```python
from build123d import *

# Parameters (mm, degrees)
EXTRUDE_1_DEPTH     = 20
OTHER_START         = 15
OTHER_1_OUTLINE_R   = 4.05
OTHER_1_DEPTH       = 20
CUT_EXTRUDE_1_DEPTH = 10


# Read off the part's stored shape, not the designer's step: 高级异型孔1
with BuildPart() as part:
    # 草图3 → 凸台-拉伸1 (new body)
    with BuildSketch(Plane.XY.offset(15)):
        with BuildLine():
            Line((26.887488657, 8.75), (45, 8.75))
            Line((45, 8.75), (45, 23.25))
            Line((45, 23.25), (26.887488657, 23.25))
            ThreePointArc((26.887488657, 23.25), (20, 26), (13.112511343, 23.25))
            Line((13.112511343, 23.25), (-5, 23.25))
            Line((-5, 23.25), (-5, 8.75))
            Line((-5, 8.75), (13.112511343, 8.75))
            ThreePointArc((13.112511343, 8.75), (20, 6), (26.887488657, 8.75))
        make_face()
    extrude(amount=EXTRUDE_1_DEPTH)

    # 高级异型孔1 outline → 高级异型孔1 (cut)
    with BuildSketch(Plane.XY.offset(OTHER_START)):
        with Locations((20, 16)):
            Circle(OTHER_1_OUTLINE_R)
    extrude(amount=OTHER_1_DEPTH, mode=Mode.SUBTRACT)

    # 草图6 → 切除-拉伸1 (cut)
    with BuildSketch(Plane.XY.offset(35)):
        with BuildLine():
            Line((-5, 15.5), (-5, 17.25))
            Line((-5, 17.25), (10, 17.25))
            Line((10, 17.25), (10, 15.5))
            Line((10, 15.5), (7, 15.5))
            ThreePointArc((7, 15.5), (6.25, 14.75), (5.5, 15.5))
            ThreePointArc((5.5, 15.5), (4.75, 16.25), (4, 15.5))
            ThreePointArc((4, 15.5), (3.25, 14.75), (2.5, 15.5))
            ThreePointArc((2.5, 15.5), (1.75, 16.25), (1, 15.5))
            ThreePointArc((1, 15.5), (0.25, 14.75), (-0.5, 15.5))
            ThreePointArc((-0.5, 15.5), (-1.25, 16.25), (-2, 15.5))
            ThreePointArc((-2, 15.5), (-2.75, 14.75), (-3.5, 15.5))
            ThreePointArc((-3.5, 15.5), (-4.25, 16.25), (-5, 15.5))
        make_face()
        with BuildLine():
            Line((45, 17.25), (30, 17.25))
            Line((30, 17.25), (30, 15.5))
            Line((30, 15.5), (33, 15.5))
            ThreePointArc((33, 15.5), (33.75, 14.75), (34.5, 15.5))
            ThreePointArc((34.5, 15.5), (35.25, 16.25), (36, 15.5))
            ThreePointArc((36, 15.5), (36.75, 14.75), (37.5, 15.5))
            ThreePointArc((37.5, 15.5), (38.25, 16.25), (39, 15.5))
            ThreePointArc((39, 15.5), (39.75, 14.75), (40.5, 15.5))
            ThreePointArc((40.5, 15.5), (41.25, 16.25), (42, 15.5))
            ThreePointArc((42, 15.5), (42.75, 14.75), (43.5, 15.5))
            ThreePointArc((43.5, 15.5), (44.25, 16.25), (45, 15.5))
            Line((45, 15.5), (45, 17.25))
        make_face()
    extrude(amount=-CUT_EXTRUDE_1_DEPTH, mode=Mode.SUBTRACT)


solid = part.part
```
Check sheet for the modelled part. Datum: model origin and axes. Units: mm. A direction names the side the tool comes from. Give positions to 0.01 mm unless a question says otherwise; leave off trailing zeros. Write each loop counter-clockwise with the first axis right and the second up, starting at its lowest first coordinate (ties: lowest second). Pieces come first, ordered by that corner, then holes.
Item 1: Cross-section at B-B (y = 12.5). Enter the section's corners in (x, z), and give its area (3 significant figures).
Item 2: Draft check along X on faces 1 (the face through (36, 8.75, 25)), 2 (the face through (20, 26, 25)), 3 (the face through (30, 16, 30)). Enter one of: released by +X, released by -X, zero draft, split by the parting line, or undercut.
Item 3: Cross-section at C-C (x = 33.75). Enter the section's corners in (y, z).
Item 4: Access from +Z, -Z, +X, -X, +Y, -Y to the whole of each face (thin tool, end or side, straight path). Record for faces 4 (the face through (2, 17.25, 30)), 5 (the face through (38, 17.25, 30)), 6 (the face through (9, 15.5, 30)), 7 (the face through (4, 8.75, 25)).
Item 5: Scan lines: L1, parallel to Y at x = 20, z = 20.5; L2, parallel to Z at x = 41, y = 17; L3, parallel to Y at x = 37.5, z = 21.5. Record each from-to range of solid material in increasing order.
Item 6: Gauge pin test, flat ends, axial feed: pin 1 (3 mm diameter, centred on x = 18, z = 27.5, fed in from +Y); pin 2 (5.5 mm diameter, centred on x = 34, z = 24.5, fed in from -Y); pin 3 (7.5 mm diameter, centred on x = 20, y = 16, fed in from -Z); pin 4 (2.5 mm diameter, centred on x = 8, z = 30, fed in from +Y). Record the tip position at first contact, or that the pin passes through.
Item 7: Cross-section at A-A (z = 18.5). Enter the section's corners in (x, y).
Report:
1. outline: (-5, 15) - (17.96, 15) - (17.96, 35) - (-5, 35) - close; (22.04, 15) - (45, 15) - (45, 35) - (22.04, 35) - close
1. area: 918 mm2
2. face 1: zero draft
2. face 2: split by the parting line
2. face 3: undercut
3. outline: (8.75, 15) - (23.25, 15) - (23.25, 35) - (17.25, 35) - (17.25, 25) - (14.75, 25) - (14.75, 35) - (8.75, 35) - close
4. face 4: +Z, -X
4. face 5: +Z, +X
4. face 6: +Z
4. face 7: +Z, -Z, -X, -Y
5. L1: y = 6 to 11.95, 20.05 to 26
5. L2: z = 15 to 25
5. L3: y = 8.75 to 23.25
6. pin 1: stops at y = 25.99
6. pin 2: stops at y = 8.75
6. pin 3: passes through
6. pin 4: stops at y = 23.25
7. outline: (-5, 8.75) - (13.11, 8.75) arc R10 ccw to (26.89, 8.75) - (45, 8.75) - (45, 23.25) - (26.89, 23.25) arc R10 ccw to (13.11, 23.25) - (-5, 23.25) - close; hole circle Ø8.1 at (20, 16)
